from build123d import *

# Parameters (mm, degrees)
EXTRUDE_THIN1_DEPTH = 22.5
SKETCH2_R           = 1.15
CUT_EXTRUDE1_DEPTH  = 88.471423905
FILLET1_R           = 1


with BuildPart() as part:
    # Sketch1 → Extrude-Thin1 (new, symmetric)
    with BuildSketch(Plane(origin=(0, 0, 0), x_dir=(0, 0, -1), z_dir=(1, 0, 0))):
        with BuildLine():
            Line((0, 0), (0, 75))
            ThreePointArc((0, 75), (-5, 80), (-10, 75))
            Line((-10, 75), (-10, 57))
            Line((-10, 57), (-13, 57))
            Line((-13, 57), (-13, 75))
            ThreePointArc((-13, 75), (-5, 83), (3, 75))
            Line((3, 75), (3, 0))
            Line((3, 0), (0, 0))
        make_face()
    extrude(amount=EXTRUDE_THIN1_DEPTH, both=True)

    # Sketch2 → Cut-Extrude1 (cut, through all)
    with BuildSketch(Plane(origin=(0, 0, -3), x_dir=(-1, 0, 0), z_dir=(0, 0, -1))):
        with Locations((-16.5, 54.245785589)):
            Circle(SKETCH2_R)
        with Locations((16.5, 54.245785589)):
            Circle(SKETCH2_R)
        with Locations((16.5, 5.745785589)):
            Circle(SKETCH2_R)
        with Locations((-16.5, 5.745785589)):
            Circle(SKETCH2_R)
    extrude(amount=-CUT_EXTRUDE1_DEPTH, mode=Mode.SUBTRACT)

    # Fillet1
    fillet1_edges = [part.edges().sort_by_distance(p)[0] for p in [
        (0, 0, -3),
        (0, 0, 0),
        (0, 57, 10),
        (0, 57, 13),
    ]]
    fillet(fillet1_edges, radius=FILLET1_R)


solid = part.part
CAD build for the part. Positions are in the model's coordinates, mm. A direction names the side the tool comes from. Coordinates: 2 decimals unless noted, no trailing zeros. Order: outer loops, then holes, each group sorted by start corner. A loop starts at its lowest first (then second) coordinate and runs counter-clockwise, first axis right, second up.
Item 1: Drill centre lines: L1, parallel to Y at x = 16.5, z = -2.3; L2, parallel to Z at x = 18.5, y = 74; L3, parallel to Y at x = -16.5, z = -0.95. Where is each one in solid material? Low to high.
Check sheet entries:
L1: y = 0.05 to 4.6, 6.9 to 53.1, 55.4 to 78.27
L2: z = -3 to 0, 10 to 13
L3: y = 0 to 4.6, 6.9 to 53.1, 55.4 to 80.35
Item 2: Band-saw the part on A-A on x = -16.5. List the corners of the cut face in (y, z), plus the area to 3 significant figures.
Check sheet entries:
outline: (0, -2) arc R1 ccw to (1, -3) - (4.6, -3) - (4.6, 0) - (1, 0) arc R1 ccw to (0, -1) - close; (6.9, -3) - (53.1, -3) - (53.1, 0) - (6.9, 0) - close; (55.4, -3) - (75, -3) arc R8 ccw to (75, 13) - (58, 13) arc R1 ccw to (57, 12) - (57, 11) arc R1 ccw to (58, 10) - (75, 10) arc R5 cw to (75, 0) - (55.4, 0) - close
area: 326 mm2
Item 3: Two-plate mould, pull along Z, no slides. Class faces 3 (the face through (22.5, 50.9, -0.4)), 4 (the face through (0, 83, 5)), 5 (the face through (0, 67, 10)): +Z half, -Z half, draft (parallel to the pull), parting line (faces both ways), or undercut.
Check sheet entries:
face 3: draft
face 4: parting line
face 5: undercut
Item 4: Band-saw the part on C-C on y = 24. List the corners of the cut face in (x, z), plus the area to 3 significant figures.
Check sheet entries:
outline: (-22.5, -3) - (22.5, -3) - (22.5, 0) - (-22.5, 0) - close
area: 135 mm2
Item 5: 3-axis set-ups, long thin cutter, end or side, ignore diameter. For faces 1 (the face through (0, 37, 0)), 2 (the face through (0, 66, 13)): which of +Z, -Z, +X, -X, +Y, -Y reach the whole face in a straight line?
Check sheet entries:
face 1: +X, -X, -Y
face 2: +Z, +X, -X, +Y, -Y
Item 6: Pin check, flat tips, straight feed: pin 1 Ø1 at (x, y) = (15, 50.5) entering from +Z; pin 2 Ø2 at (x, z) = (0, 9) entering from +Y; pin 3 Ø0.8 at (x, z) = (10, 11.5) entering from -Y. Stop position of each tip, or through.
Check sheet entries:
pin 1: stops at z = 0
pin 2: stops at y = 82.42
pin 3: stops at y = 57
Item 7: Band-saw the part on B-B on z = 5. List the corners of the cut face in (x, y).
Check sheet entries:
outline: (-22.5, 80) - (22.5, 80) - (22.5, 83) - (-22.5, 83) - close
